Source: three-view drawing plus pictorial views. Frame: mm from the lowest corner of the part. Give positions to 0.01 mm unless a question says otherwise; leave off trailing zeros. Order: outer loops, then holes, each group sorted by start corner. A loop starts at its lowest first (then second) coordinate and runs counter-clockwise, first axis right, second up. Notation, with made-up numbers: M 84.25,-23.75 L 139.25,-23.75 A26 ccw 139.25,-1.75 Z; hole C -0.75,-18 d9. An arc over 180 degrees is marked long. Use CSV: the item, a comma, the result in double quotes. Start each with the question number.
Item 1: Section query A-A on z = 27.25. Return loops of the section in (x, y).
Item 2: Ray query, probe 1 along Z at (x, y) = (3.2, 1.1); probe 2 along X at (y, z) = (0.5, 27.25); probe 3 along X at (y, z) = (1.45, 53.5). Return the intervals inside material, ascending. Write a range as from..to.
Item 3: First-contact query: pin 1 (3 mm diameter, centred on x = 3.2, z = 27.25, fed in from -Y). Flat tip, straight axial feed; report the tip coordinate or a pass-through.
Item 4: Section query B-B on y = 0.65. Return loops of the section in (x, z).
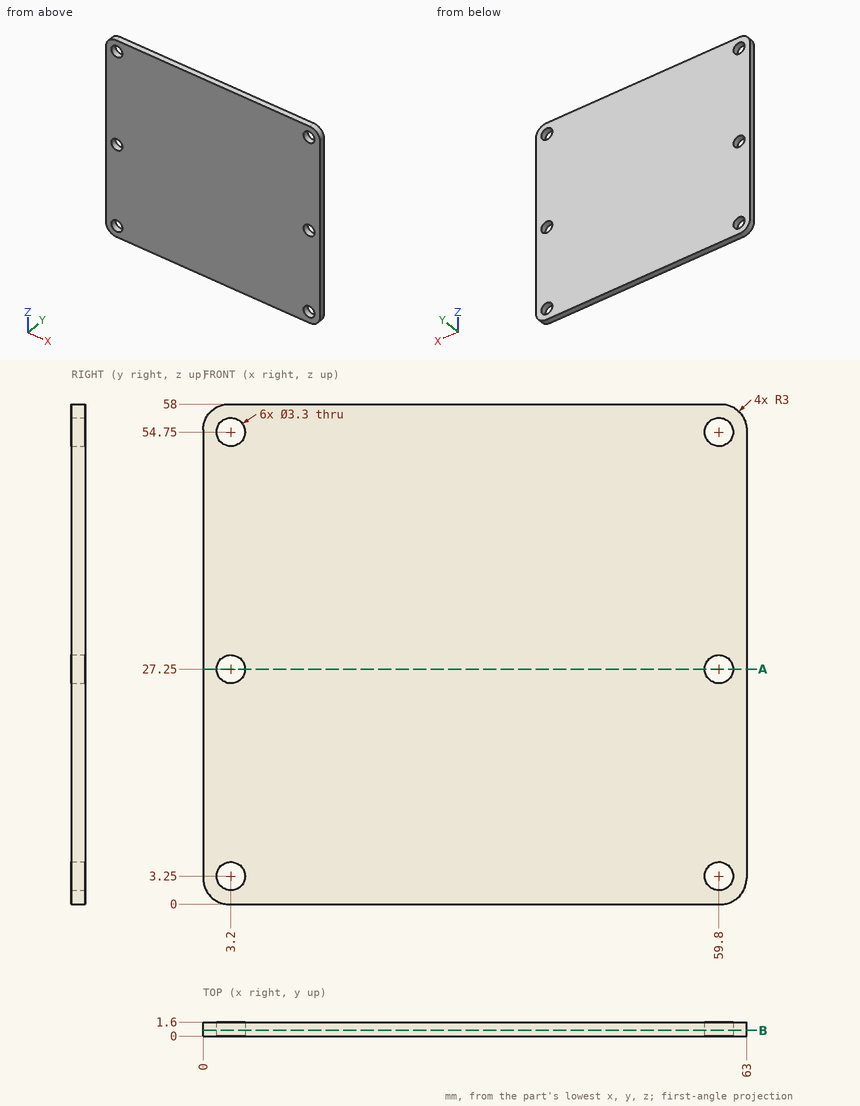
Verdict:
1,outline,"M 0,0 L 1.55,0 L 1.55,1.6 L 0,1.6 Z; M 4.85,0 L 58.15,0 L 58.15,1.6 L 4.85,1.6 Z; M 61.45,0 L 63,0 L 63,1.6 L 61.45,1.6 Z"
2,probe 1,"0..1.6, 4.9..25.6, 28.9..53.1, 56.4..58"
2,probe 2,"0..1.55, 4.85..58.15, 61.45..63"
2,probe 3,"0..2.12, 4.28..58.72, 60.88..63"
3,pin 1,"through"
4,outline,"M 0,3 A3 ccw 3,0 L 60,0 A3 ccw 63,3 L 63,55 A3 ccw 60,58 L 3,58 A3 ccw 0,55 Z; hole C 3.2,3.25 d3.3; hole C 3.2,27.25 d3.3; hole C 3.2,54.75 d3.3; hole C 59.8,3.25 d3.3; hole C 59.8,27.25 d3.3; hole C 59.8,54.75 d3.3"
